Check sheet for the modelled part. Datum: model origin and axes. Units: mm. Round coordinates to 2 decimals unless told otherwise and drop trailing zeros. Write each loop counter-clockwise with the first axis right and the second up, starting at its lowest first coordinate (ties: lowest second). Pieces come first, ordered by that corner, then holes. Notation, with made-up numbers: (-22, 0) - (30, 0) arc R16 ccw to (30, 11) - close; hole circle Ø4 at (-9, 74.25). An arc over 180 degrees is marked (long way). Answer as a JSON object with one key per item and string values. Group by question number.
Item 1: Gauge pin test, flat end, axial feed: P1, Ø4.5, axis at x = 40, y = 0, coming from the -Z side. Record the tip position at first contact, or that the pin passes through.
Item 2: Thickness scan on line 1 (X direction, y = 0.5, z = 1.75); line 2 (Y direction, x = 40, z = 2.05); line 3 (X direction, y = 0.75, z = 2.25). Record the ranges inside material, lowest first.
Item 3: Sectioned sample at A-A on y = 0. Record the boundary of the cut face in (x, z), plus the area to 3 significant figures.
Item 4: Sectioned sample at B-B on z = 1.65. Record the boundary of the cut face in (x, y), plus the area to 3 significant figures.
```python
from build123d import *

# Parameters (mm, degrees)
SKETCH1_R           = 4
SKETCH1_W           = 80
SKETCH1_H           = 8
BOSS_EXTRUDE1_DEPTH = 3
SKETCH2_R           = 2.5
CUT_EXTRUDE1_DEPTH  = 3


with BuildPart() as part:
    # Sketch1 → Boss-Extrude1 (new body)
    with BuildSketch(Plane.XY):
        with Locations((-40, 0)):
            Circle(SKETCH1_R)
        with Locations((40, 0)):
            Circle(SKETCH1_R)
        Rectangle(SKETCH1_W, SKETCH1_H)
    extrude(amount=BOSS_EXTRUDE1_DEPTH)

    # Sketch2 → Cut-Extrude1 (cut)
    with BuildSketch(Plane.XY.offset(3)):
        with Locations((-40, 0)):
            Circle(SKETCH2_R)
        with Locations((40, 0)):
            Circle(SKETCH2_R)
    extrude(amount=-CUT_EXTRUDE1_DEPTH, mode=Mode.SUBTRACT)


solid = part.part
```
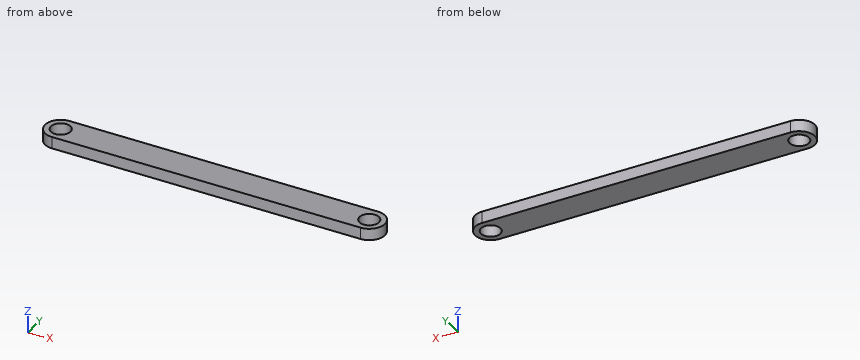
Completed:
{
 "1": {"P1": "through"},
 "2": {"line 1": "-43.97 to -42.45, -37.55 to 37.55, 42.45 to 43.97", "line 2": "-4 to -2.5, 2.5 to 4", "line 3": "-43.93 to -42.38, -37.62 to 37.62, 42.38 to 43.93"},
 "3": {"outline": "(-44, 0) - (-42.5, 0) - (-42.5, 3) - (-44, 3) - close; (-37.5, 0) - (37.5, 0) - (37.5, 3) - (-37.5, 3) - close; (42.5, 0) - (44, 0) - (44, 3) - (42.5, 3) - close", "area": "234 mm²"},
 "4": {"outline": "(-40, -4) - (40, -4) arc R4 ccw to (40, 4) - (-40, 4) arc R4 ccw to start; hole circle Ø5 at (-40, 0); hole circle Ø5 at (40, 0)", "area": "651 mm²"}
}
